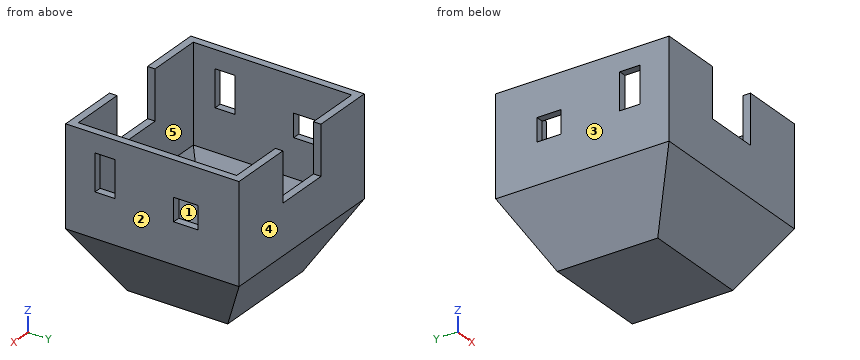
```python
from build123d import *

# Parameters (mm, degrees)
F0_W      = 87.4929502606
F0_H      = 80.8734223247
F1_DEPTH  = 50.8
F1_TAPER  = -30
F3_W      = 88.9319777489
F3_H      = 89.219789952
F2_W      = 146.1517376103
F2_H      = 139.5322096743
F4_DEPTH  = 79.502
F6_SCALE  = 0.21
F7_T      = -1.27
F8_W      = 4.72650351
F8_H      = 8.3095808529
F8_W_2    = 4.5930747874
F9_DEPTH  = 29.3027641316
F10_W     = 3.3891107887
F10_H     = 6.2133707106
F10_W_2   = 4.0794850793
F10_H_2   = 3.8912016898
F11_DEPTH = 30.6928649982


with BuildPart() as f1:
    # F0 (on Top) → F1 (new body)
    with BuildSketch(Plane.XY):
        with Locations((0, -0.7195137441)):
            Rectangle(F0_W, F0_H)
    extrude(amount=F1_DEPTH, taper=F1_TAPER)

    # F3 (on face) + F2 (on face) → F4 (join)
    with BuildSketch(Plane.XY.offset(50.8)):
        with Locations((1.0073184967, -1.4390293509)):
            Rectangle(F3_W, F3_H)
    with BuildSketch(Plane.XY.offset(50.8)):
        with Locations((0, -0.7195137441)):
            Rectangle(F2_W, F2_H)
    extrude(amount=F4_DEPTH)


with BuildPart() as f1_1:
    # F6: moved
    add(f1.part.scale(F6_SCALE))

    # F7
    f7_openings = [f1_1.faces().sort_by_distance(p)[0] for p in [
        (0, -0.151098, 27.36342),
    ]]
    offset(amount=F7_T, openings=f7_openings)

    # F8 (on face) → F9 (cut, through all)
    with BuildSketch(Plane.XZ.offset(14.8019799021)):
        with Locations((-2.363251755, 23.2086295735)):
            Rectangle(F8_W, F8_H)
        with Locations((2.2965373937, 23.2086295735)):
            Rectangle(F8_W_2, F8_H)
    extrude(amount=-F9_DEPTH, mode=Mode.SUBTRACT)

    # F10 (on face) → F11 (cut, through all)
    with BuildSketch(Plane(origin=(-15.3459324491, 0, 0), x_dir=(0, -1, 0), z_dir=(-1, 0, 0))):
        with Locations((8.1630637869, 21.1822334677)):
            Rectangle(F10_W, F10_H)
        with Locations((-5.4875212954, 19.4562980905)):
            Rectangle(F10_W_2, F10_H_2)
    extrude(amount=-F11_DEPTH, mode=Mode.SUBTRACT)


solid = f1_1.part
```
Input: part model. Units: mm. Frame: model coordinates. Face numbers are marked on the shaded views. A direction names the side the tool comes from. Round coordinates to 2 decimals unless told otherwise and drop trailing zeros. Write each loop counter-clockwise with the first axis right and the second up, starting at its lowest first coordinate (ties: lowest second). Pieces come first, ordered by that corner, then holes. Notation, with made-up numbers: M 75.5,-14.75 L 84.5,-14.75 A30 cw 84.5,8.25 Z; hole C 7,-39 d11. An arc over 180 degrees is marked long. Write each question's results on one line, items separated by ' | '.
Q1. Pin query (flat end, axial travel): P1, Ø3, axis at x = 9, y = -10.5, coming from the +Z side; P2, Ø1.5, axis at x = 3, z = 4, coming from the -Y side; P3, Ø0.6, axis at x = 14.5, y = -8, coming from the -Z side. Return the tip coordinate at first contact, or that it passes through.
Results:
P1: stops at z = 8.35 | P2: stops at y = -11.39 | P3: stops at z = 8.68
Q2. Section query A-A (z = 11.75). Return loops of the section in (x, y), and give its area (3 significant figures).
Results:
outline: M -15.35,-14.8 L 15.35,-14.8 L 15.35,14.5 L -15.35,14.5 Z; hole M -14.08,-13.53 L 14.08,-13.53 L 14.08,13.23 L -14.08,13.23 Z | area: 146 mm^2
Q3. Draft query along X for the marked faces 1, 2 and 3. Return one class per face: released by +X, released by -X, zero draft, split by the parting line, or undercut.
Results:
face 1: undercut | face 2: released by +X | face 3: released by -X
Q4. Section query C-C (y = 4). State how many separate pieces and enclosed holes the cut face has, and give its area (3 significant figures).
Results:
separate pieces: 3 | enclosed holes: 0 | area: 84.4 mm^2
Q5. Line query: line 1 along Y through (x, z) = (-1.5, 14.75); line 2 along X through (y, z) = (13, 21); line 3 along X through (y, z) = (0.5, 4.5). Output: solid intervals per line, ascending.
Results:
line 1: y = -14.8 to -13.53, 13.23 to 14.5 | line 2: x = -15.35 to -14.08, 14.08 to 15.35 | line 3: x = -11.78 to -10.32, 10.32 to 11.78
Q6. Section query B-B (z = 23.5). Return loops of the section in (x, y).
Results:
outline: M -15.35,-14.8 L -4.73,-14.8 L -4.73,-13.53 L -14.08,-13.53 L -14.08,-9.86 L -15.35,-9.86 Z; M -15.35,-6.47 L -14.08,-6.47 L -14.08,13.23 L -4.73,13.23 L -4.73,14.5 L -15.35,14.5 Z; M 4.59,-14.8 L 15.35,-14.8 L 15.35,-9.86 L 14.08,-9.86 L 14.08,-13.53 L 4.59,-13.53 Z; M 4.59,13.23 L 14.08,13.23 L 14.08,-6.47 L 15.35,-6.47 L 15.35,14.5 L 4.59,14.5 Z
Q7. Access query for the marked faces 4 and 5. Directions: +Z, -Z, +X, -X, +Y, -Y. A direction counts if a zero-diameter tool reaches every point of the face in a straight line with its end or side. Return the directions, or none.
Results:
face 4: +Z, -Z, +X, -X, +Y | face 5: +Z
